For this review, take the finished solid that the model builds, in its own axes (mm). Face numbers are marked on the shaded views. A direction names the side the tool comes from. Round coordinates to 2 decimals unless told otherwise and drop trailing zeros. Order: outer loops, then holes, each group sorted by start corner. A loop starts at its lowest first (then second) coordinate and runs counter-clockwise, first axis right, second up. Notation, with made-up numbers: (20.25, 38.25) -> (54.25, 38.25) arc R17 cw to (54.25, 68.25) -> close; hole circle Ø1 at (41, 13). An arc over 180 degrees is marked (long way). Put each result on its own line as item: value. Start each with the question number.
```python
from build123d import *

# Parameters (mm, degrees)
SKETCH1_W           = 12.7
SKETCH1_H           = 25.4
BOSS_EXTRUDE1_DEPTH = 21.082
SKETCH3_W           = 8.128
SKETCH3_H           = 13.208
CUT_EXTRUDE2_DEPTH  = 27.94
SKETCH4_W           = 5.08
SKETCH4_H           = 5.334
CUT_EXTRUDE3_DEPTH  = 27.94
SKETCH5_W           = 12.7
SKETCH5_H           = 21.082
BOSS_EXTRUDE2_DEPTH = 2.54


with BuildPart() as part:
    # Sketch1 → Boss-Extrude1 (new body)
    with BuildSketch(Plane.XY):
        Rectangle(SKETCH1_W, SKETCH1_H)
    extrude(amount=BOSS_EXTRUDE1_DEPTH)

    # Sketch3 → Cut-Extrude2 (cut)
    with BuildSketch(Plane(origin=(0, 12.7, 0), x_dir=(1, 0, 0), z_dir=(0, 1, 0))):
        with Locations((0, -11.938)):
            Rectangle(SKETCH3_W, SKETCH3_H)
    extrude(amount=-CUT_EXTRUDE2_DEPTH, mode=Mode.SUBTRACT)

    # Sketch4 → Cut-Extrude3 (cut)
    with BuildSketch(Plane(origin=(0, 12.7, 0), x_dir=(1, 0, 0), z_dir=(0, 1, 0))):
        with Locations((-1.524, -2.667)):
            Rectangle(SKETCH4_W, SKETCH4_H)
    extrude(amount=-CUT_EXTRUDE3_DEPTH, mode=Mode.SUBTRACT)

    # Sketch5 → Boss-Extrude2 (add)
    with BuildSketch(Plane(origin=(0, 12.7, 0), x_dir=(1, 0, 0), z_dir=(0, 1, 0))):
        with Locations((0, -10.541)):
            Rectangle(SKETCH5_W, SKETCH5_H)
    extrude(amount=BOSS_EXTRUDE2_DEPTH)


solid = part.part
```
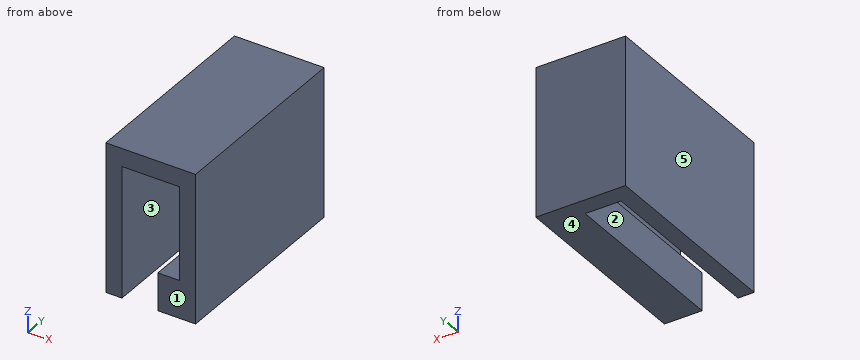
Item 1: Consider section B-B, the plane x = -1.5. Write out the cut boundary in (y, z).
Item 2: Insertion check: pin 1 Ø2.5 at (x, y) = (-1.5, -4.5) entering from -Z; pin 2 Ø2 at (x, z) = (-2.5, 8) entering from -Y. Each pin has a flat end and moves straight along its axis. Give the tip position at first contact, or say it passes through.
Item 3: Consider section A-A, the plane y = 1.5. Write out the cut boundary in (x, z).
Item 4: Tool access review of the marked faces 1 and 2: name each direction out of +Z, -Z, +X, -X, +Y, -Y from which nothing blocks a thin tool from reaching the whole face with its end or side.
Item 5: Consider section D-D, the plane x = 3.5. Write out the cut boundary in (y, z), plus the area to 3 significant figures.
Item 6: For L1, parallel to Z at x = 1.25, y = 10.5; L2, parallel to X at y = 3, z = 8.5; L3, parallel to X at y = -1, z = 3, list the stretches that pass through material, from the lowest coordinate up.
Item 7: Consider section C-C, the plane z = 11. Write out the cut boundary in (x, y), plus the area to 3 significant figures.
Item 8: Mouldability with a two-part tool opening along X and no side actions: class the marked faces 3, 4 and 5 as +X half, -X half, draft (parallel to the pull), parting line (faces both ways), or undercut.
Evaluation:
1. outline: (-12.7, 18.54) -> (12.7, 18.54) -> (12.7, 0) -> (15.24, 0) -> (15.24, 21.08) -> (-12.7, 21.08) -> close
2. pin 1: stops at z = 18.54
2. pin 2: stops at y = 12.7
3. outline: (-6.35, 0) -> (-4.06, 0) -> (-4.06, 18.54) -> (4.06, 18.54) -> (4.06, 5.33) -> (1.02, 5.33) -> (1.02, 0) -> (6.35, 0) -> (6.35, 21.08) -> (-6.35, 21.08) -> close
4. face 1: +Z, -Z, +X, -X, -Y
4. face 2: -Z, -Y
5. outline: (-12.7, 0) -> (15.24, 0) -> (15.24, 21.08) -> (-12.7, 21.08) -> (-12.7, 18.54) -> (12.7, 18.54) -> (12.7, 5.33) -> (-12.7, 5.33) -> close
5. area: 254 mm^2
6. L1: z = 0 to 5.33, 18.54 to 21.08
6. L2: x = -6.35 to -4.06, 4.06 to 6.35
6. L3: x = -6.35 to -4.06, 1.02 to 6.35
7. outline: (-6.35, -12.7) -> (-4.06, -12.7) -> (-4.06, 12.7) -> (4.06, 12.7) -> (4.06, -12.7) -> (6.35, -12.7) -> (6.35, 15.24) -> (-6.35, 15.24) -> close
7. area: 148 mm^2
8. face 3: undercut
8. face 4: draft
8. face 5: -X half
